Geometry check sheet. Reference: the model listing, model coordinates, mm. A direction names the side the tool comes from. Coordinates: 2 decimals unless noted, no trailing zeros. Write each loop counter-clockwise with the first axis right and the second up, starting at its lowest first coordinate (ties: lowest second). Pieces come first, ordered by that corner, then holes. Notation, with made-up numbers: M 55,43 L 61,43 A16 ccw 61,50 Z; hole C 35.5,54.25 d2. An arc over 180 degrees is marked long. Write item = value, one per line. Start each with the question number.
```python
from build123d import *

# Parameters (mm, degrees)
F0_W     = 40
F0_H     = 40
F1_DEPTH = 145
F0_W_2   = 630
F0_H_2   = 550
F2_DEPTH = 40


with BuildPart() as f1:
    # F0 (on Top) → F1 (new body)
    with BuildSketch(Plane.XY):
        with Locations((-335, 295)):
            Rectangle(F0_W, F0_H)
    extrude(amount=-F1_DEPTH)



with BuildPart() as f1b:
    # F0 (on Top) → F1, piece 2 (new body)
    with BuildSketch(Plane.XY):
        with Locations((335, 295)):
            Rectangle(F0_W, F0_H)
    extrude(amount=-F1_DEPTH)


with BuildPart() as f1c:
    # F0 (on Top) → F1, piece 3 (new body)
    with BuildSketch(Plane.XY):
        with Locations((335, -295)):
            Rectangle(F0_W, F0_H)
    extrude(amount=-F1_DEPTH)


with BuildPart() as f1d:
    # F0 (on Top) → F1, piece 4 (new body)
    with BuildSketch(Plane.XY):
        with Locations((-335, -295)):
            Rectangle(F0_W, F0_H)
    extrude(amount=-F1_DEPTH)


with BuildPart() as f1_1:
    add(f1.part)

    add(f1b.part)  # F2 merges F1b

    add(f1c.part)  # F2 merges F1c

    add(f1d.part)  # F2 merges F1d
    # F0 (on Top) → F2 (join)
    with BuildSketch(Plane.XY):
        with Locations((0, -295)):
            Rectangle(F0_W_2, F0_H)
        with Locations((335, 0)):
            Rectangle(F0_W, F0_H_2)
        with Locations((0, 295)):
            Rectangle(F0_W_2, F0_H)
        with Locations((-335, 0)):
            Rectangle(F0_W, F0_H_2)
    extrude(amount=-F2_DEPTH)


solid = f1_1.part
```
Q1. Scan lines: L1, parallel to X at y = 254, z = -8.5; L2, parallel to Y at x = 326, z = -98.5; L3, parallel to Z at x = 325, y = 67. Record each from-to range of solid material in increasing order.
Q2. Cross-section at A-A on y = 145. Enter the section's corners in (x, z).
Q3. Set-up check for faces 4 (the face through (335, -275, -92)), 5 (the face through (315, -4, -20)), 6 (the face through (-4, -295, -40)): record each of +Z, -Z, +X, -X, +Y, -Y from which the full face is reachable in a straight line by a thin tool's end or side.
Q4. Cross-section at B-B on x = 258. Enter the section's corners in (y, z), and give its area (3 significant figures).
Q5. Draft check along Y on faces 1 (the face through (335, 275, -92)), 2 (the face through (-315, -4, -20)), 3 (the face through (-335, 295, -145)). Enter one of: pulls with the +Y half, pulls with the -Y half, needs draft (parallel to the pull), parting line crosses it, or undercut.
Q6. Cross-section at C-C on z = -75.5. Enter the section's corners in (x, y), and give its area (3 significant figures).
Q7. Cross-section at D-D on z = -14.5. Enter the section's corners in (x, y).
Q8. Gauge pin test, flat end, axial feed: pin 1 (12 mm diameter, centred on x = 61, y = 298.5, fed in from -Z). Record the tip position at first contact, or that the pin passes through.
Values found:
q1.L1 = -355 to -315, 315 to 355
q1.L2 = -315 to -275, 275 to 315
q1.L3 = -40 to 0
q2.outline = M -355,-40 L -315,-40 L -315,0 L -355,0 Z; M 315,-40 L 355,-40 L 355,0 L 315,0 Z
q3.face_4 = -Z, +X, -X
q3.face_5 = +Z, -Z
q3.face_6 = -Z, +Y, -Y
q4.outline = M -315,-40 L -275,-40 L -275,0 L -315,0 Z; M 275,-40 L 315,-40 L 315,0 L 275,0 Z
q4.area = 3,200 mm²
q5.face_1 = undercut
q5.face_2 = undercut
q5.face_3 = needs draft
q6.outline = M -355,-315 L -315,-315 L -315,-275 L -355,-275 Z; M -355,275 L -315,275 L -315,315 L -355,315 Z; M 315,-315 L 355,-315 L 355,-275 L 315,-275 Z; M 315,275 L 355,275 L 355,315 L 315,315 Z
q6.area = 6,400 mm²
q7.outline = M -355,-315 L 355,-315 L 355,315 L -355,315 Z; hole M -315,-275 L 315,-275 L 315,275 L -315,275 Z
q8.pin_1 = -40
